Job drawing, mm, ordinate dimensions from the low corner. One solid piece. A direction names the side the tool comes from. Round coordinates to 2 decimals unless told otherwise and drop trailing zeros. Loops run counter-clockwise (first coordinate to the right, second up) from the corner with the lowest first, then second, coordinate; pieces in that order, holes last. Notation, with made-up numbers: M 65.5,-26.75 L 76.5,-26.75 A20 cw 76.5,-5.75 Z; hole C -31.75,-2 d11. An arc over 180 degrees is marked long. One line per item, written item: value.
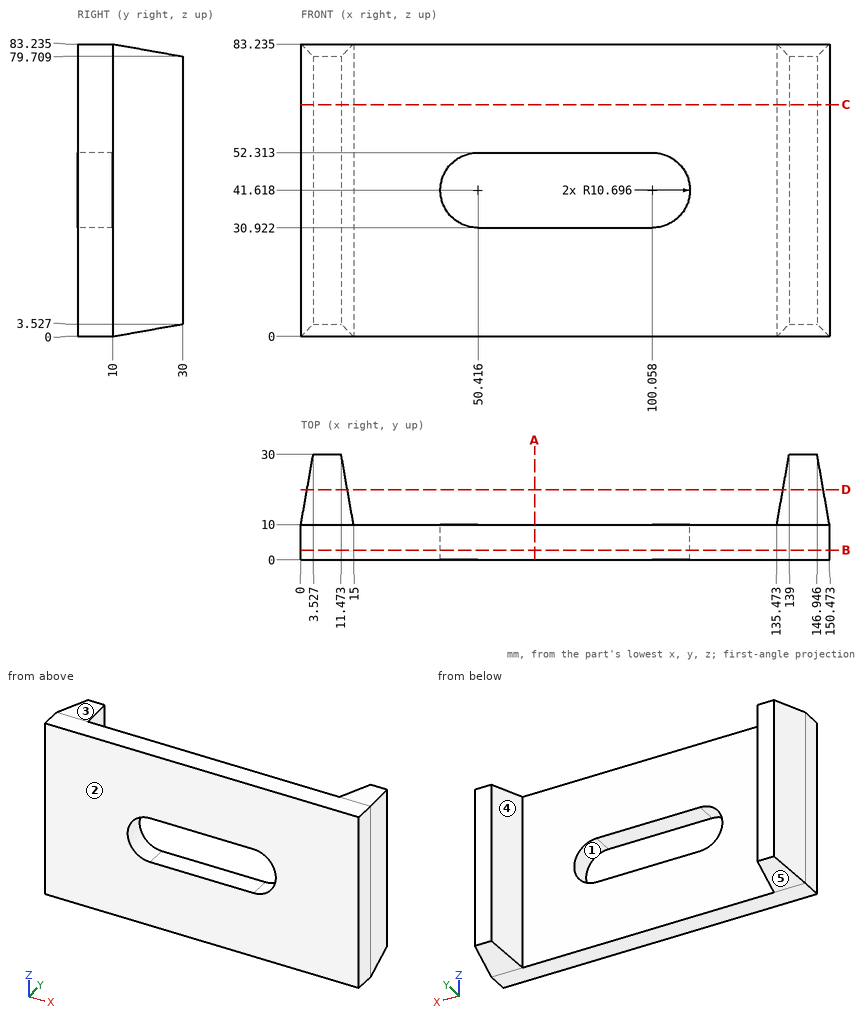
Item 1: Slice it at C-C, the plane z = 66. Give the cut face in (x, y), and give its area (3 significant figures).
Check values:
outline: M 0,0 L 150.47,0 L 150.47,10 L 146.95,30 L 139,30 L 135.47,10 L 15,10 L 11.47,30 L 3.53,30 L 0,10 Z
area: 1,960 mm2
Item 2: Wall check: line 1 along Z through (x, y) = (88, 5.75) (1 decimal); line 2 along X through (y, z) = (8.5, 42); line 3 along Y through (x, z) = (80.5, 72). Give the ranges that are in metal, low to high.
Check values:
line 1: z = 0 to 30.9, 52.3 to 83.2
line 2: x = 0 to 39.73, 110.75 to 150.47
line 3: y = 0 to 10
Item 3: Slice it at B-B, the plane y = 2.75. Give the cut face in (x, z) (1 decimal).
Check values:
outline: M 0,0 L 150.5,0 L 150.5,83.2 L 0,83.2 Z; hole M 50.4,30.9 L 100.1,30.9 A10.7 ccw 100.1,52.3 L 50.4,52.3 A10.7 ccw Z
Item 4: Slice it at D-D, the plane y = 20. Give the cut face in (x, z), and give its area (3 significant figures).
Check values:
outline: M 1.76,1.76 L 13.24,1.76 L 13.24,81.47 L 1.76,81.47 Z; M 137.24,1.76 L 148.71,1.76 L 148.71,81.47 L 137.24,81.47 Z
area: 1,830 mm2
Item 5: Which spindle directions (+Z, -Z, +X, -X, +Y, -Y) get a long thin tool onto all of the face, cutting with end or side? Do the marked faces 4 and 5. Say none if no direction does.
Check values:
face 4: +Z, -Z, +Y
face 5: -Z, +X, -X, +Y
Item 6: Slice it at A-A, the plane x = 66.5. Give the cut face in (y, z) (1 decimal).
Check values:
outline: M 0,0 L 10,0 L 10,30.9 L 0,30.9 Z; M 0,52.3 L 10,52.3 L 10,83.2 L 0,83.2 Z
Item 7: Pull direction Z, two halves, no side cores. Call the marked faces 1, 2 and 3: pulls with the +Z half, pulls with the -Z half, needs draft (parallel to the pull), parting line crosses it, or undercut.
Check values:
face 1: undercut
face 2: needs draft
face 3: pulls with the +Z half
Item 8: Drop flat-ended pins along their axis: P1, Ø8, axis at x = 133.5, y = 19.5, coming from the +Z side (1 decimal); P2, Ø2, axis at x = 32.5, z = 62, coming from the +Y side. Give the stop position or say it passes through.
Check values:
P1: stops at z = 82
P2: stops at y = 10
